Read the model definition and answer for the solid it produces. Units are mm, in the model's axes. Round coordinates to 2 decimals unless told otherwise and drop trailing zeros. Loops run counter-clockwise (first coordinate to the right, second up) from the corner with the lowest first, then second, coordinate; pieces in that order, holes last. Notation, with made-up numbers: (59, 12.5) - (107, 12.5) arc R27 ccw to (107, 33.5) - close; hole circle Ø6 at (-14, -16). An arc over 180 degrees is marked (long way). Answer as CSV lines item,"result".
```python
from build123d import *

# Parameters (mm, degrees)
ESBO_O1_R                = 2.5
RESSALTO_EXTRUS_O1_DEPTH = 65
ESBO_O2_W                = 7.122508342
ESBO_O2_H                = 3.466033472
CORTE_EXTRUS_O1_DEPTH    = 130


with BuildPart() as part:
    # Esboço1 → Ressalto-extrusão1 (new, symmetric)
    with BuildSketch(Plane.YZ):
        with Locations(Location((0, 0, 0), (0, 0, 270))):
            Circle(ESBO_O1_R)
    extrude(amount=RESSALTO_EXTRUS_O1_DEPTH, both=True)

    # Esboço2 → Corte-extrusão1 (cut)
    with BuildSketch(Plane.YZ.offset(65)):
        with Locations((0.399926939, 3.733016736)):
            Rectangle(ESBO_O2_W, ESBO_O2_H)
    corte_extrus_o1 = extrude(amount=-CORTE_EXTRUS_O1_DEPTH, mode=Mode.SUBTRACT)

    # Espelhar1: Corte-extrusão1 across plane
    add(corte_extrus_o1.mirror(Plane.XY), mode=Mode.SUBTRACT)


solid = part.part
```
1) A cutting plane is placed at B-B, the plane z = 1.1. Determine the outline of the cut face in (x, y) (3 decimals), plus the area to 3 significant figures.
Entries:
outline,"(-65, -2.245) - (65, -2.245) - (65, 2.245) - (-65, 2.245) - close"
area,"584 mm^2"
2) Find the intervals of material crossed by line 1 (Y direction, x = -43.5, z = -0.25); line 2 (Y direction, x = -3, z = 1.25); line 3 (Z direction, x = -39, y = 1.85), in increasing order.
Entries:
line 1,"y = -2.49 to 2.49"
line 2,"y = -2.17 to 2.17"
line 3,"z = -1.68 to 1.68"
3) A cutting plane is placed at A-A, the plane x = 16. Determine the outline of the cut face in (y, z), plus the area to 3 significant figures.
Entries:
outline,"(-1.5, -2) - (1.5, -2) arc R2.5 ccw to (1.5, 2) - (-1.5, 2) arc R2.5 ccw to start"
area,"17.6 mm^2"
